Model file for the job. Use its own axes, mm. Round coordinates to 2 decimals unless told otherwise and drop trailing zeros. Order: outer loops, then holes, each group sorted by start corner. A loop starts at its lowest first (then second) coordinate and runs counter-clockwise, first axis right, second up. Notation, with made-up numbers: (65.25, 69) - (122.25, 69) arc R13 cw to (122.25, 94) - close; hole circle Ø1 at (-0.5, 52.5). An arc over 180 degrees is marked (long way). Write item = value, one per line.
Autodesk Fusion 360 part; units mm, degrees
sketch "Sketch1" plane through (0, 0, 0) normal (0, 0, 1) x (1, 0, 0)
  spline S0 degree 5 poles (0, 0.083) (3.4028, 0.6487) (10.1655, 1.6592) (20.1813, 2.8133) (33.3011, 3.6916) (49.3449, 3.7981) (61.865, 3.0163) (71.0307, 1.8175) (77.0289, 0.7123) (80, 0.083) knots 0 0 0 0 0 0 0.2 0.4 0.6 0.8 1 1 1 1 1 1
  line L0 (72.4946, 1.6726) -> (87.5054, -1.5065)
  line L1 (-8.6308, -1.3517) -> (8.6308, 1.5177)
  spline S1 degree 5 poles (0, 17.083) (3.4028, 16.5174) (10.1655, 15.5068) (20.1813, 14.3528) (33.3011, 13.4745) (49.3449, 13.368) (61.865, 14.1497) (71.0307, 15.3485) (77.0289, 16.4538) (80, 17.083) knots 0 0 0 0 0 0 0.2 0.4 0.6 0.8 1 1 1 1 1 1
  line L2 (-8.6308, 18.5177) -> (8.6308, 15.6483)
  line L3 (72.4946, 15.4935) -> (87.5054, 18.6726)
  line L4 (80, 17.083) -> (80, 0.083)
  line L5 (0, 17.083) -> (0, 0.083)
  circle A0 centre (40, 8.5) radius 2.6
  dimension "d13" = 5.2
  dimension "d14" = 40
  dimension "d15" = 40
  dimension "d18" = 17
  dimension "d21" = 17
  dimension "d22" = 8.5
extrude "Extrude4" add sketch "Sketch1" along normal blind 4
extrude "Extrude2" [suppressed]
extrude "Extrude3" [suppressed]
equation "d22 = ( 17 / 2 ) * 1 mm"
1) Cut at A-A (y = 8.5). Write the cut outline in (x, z).
Conclusion:
outline = (0, 0) - (37.4, 0) - (37.4, 4) - (0, 4) - close; (42.6, 0) - (80, 0) - (80, 4) - (42.6, 4) - close
2) Wall check: line 1 along Y through (x, z) = (40, 2.55); line 2 along X through (y, z) = (10, 0.7); line 3 along X through (y, z) = (6.5, 0.85). Give the ranges that are in metal, low to high.
Conclusion:
line_1 = 3.6 to 5.9, 11.1 to 13.56
line_2 = 0 to 37.88, 42.12 to 80
line_3 = 0 to 38.34, 41.66 to 80
3) Mould opens along X. For faces 1 (the face through (80, 9, 2)), 2 (the face through (0, 9, 2)), 3 (the face through (39, 5, 0)), 4 (the face through (37.4, 8.4, 2)) say: +X half, -X half, draft (parallel to the pull), parting line (faces both ways), or undercut.
Conclusion:
face_1 = +X half
face_2 = -X half
face_3 = draft
face_4 = undercut
